CAD build for the part. Positions are in the model's coordinates, mm. A direction names the side the tool comes from. Coordinates: 2 decimals unless noted, no trailing zeros. Write each loop counter-clockwise with the first axis right and the second up, starting at its lowest first coordinate (ties: lowest second). Pieces come first, ordered by that corner, then holes. Notation, with made-up numbers: M 60,48 L 67,48 A16 ccw 67,78 Z; hole C -31.75,67 d2. An arc over 180 degrees is marked long. Put each result on its own line as item: value. Start each with the question number.
```python
from build123d import *

# Parameters (mm, degrees)
F0_R          = 13
F1_DEPTH      = 6
F2_R          = 10.5
F3_DEPTH      = 19
F3_DEPTH_BACK = 110
F6_START      = -19
F5_R          = 11.5
F5_R_2        = 10.5
F6_DEPTH      = 3
F8_START      = -15
F7_R          = 12.5
F7_R_2        = 10.5
F8_DEPTH      = 4
F10_DEPTH     = 5
F11_R         = 4.5
F12_DEPTH     = 153


with BuildPart() as f1:
    # F0 (on Front) → F1 (new body)
    with BuildSketch(Plane.XZ):
        Circle(F0_R)
    extrude(amount=F1_DEPTH)

    # F2 (on face) → F3 (join, two sides)
    with BuildSketch(Plane.XZ.offset(6)) as f3_sk:
        Circle(F2_R)
    extrude(amount=F3_DEPTH)
    extrude(f3_sk.sketch, amount=-F3_DEPTH_BACK)

    # F5 (on face) → F6 (join)
    with BuildSketch(Plane(origin=(0, 104, 0), x_dir=(-1, 0, 0), z_dir=(0, 1, 0)).offset(F6_START)):
        Circle(F5_R)
        Circle(F5_R_2, mode=Mode.SUBTRACT)
    extrude(amount=-F6_DEPTH)

    # F7 (on face) → F8 (join)
    with BuildSketch(Plane(origin=(0, 104, 0), x_dir=(-1, 0, 0), z_dir=(0, 1, 0)).offset(F8_START)):
        Circle(F7_R)
        Circle(F7_R_2, mode=Mode.SUBTRACT)
    extrude(amount=-F8_DEPTH)

    # F9 (on face) → F10 (join)
    with BuildSketch(Plane.XZ.offset(25)):
        Polygon((9.3875564858, -3.3022610956), (7.5536202416, 6.4787318484), (-1.8339362442, 9.780992944), (-9.3875564858, 3.3022610956), (-7.5536202416, -6.4787318484), (1.8339362442, -9.780992944), align=None)
    extrude(amount=F10_DEPTH)

    # F11 (on face) → F12 (cut)
    with BuildSketch(Plane.XZ.offset(30)):
        Circle(F11_R)
    extrude(amount=-F12_DEPTH, mode=Mode.SUBTRACT)


solid = f1.part
```
(1) Slice it at B-B, the plane y = 66.5. Write the cut outline in (x, z).
(2) Two-plate mould, pull along Y, no slides. Class faces 5 (the face through (4.04, -30, 2.31)), 6 (the face through (-3.4, 82, -10.2)), 7 (the face through (-10.316, -2.958, -7.91)): +Y half, -Y half, draft (parallel to the pull), parting line (faces both ways), or undercut.
(3) Which spindle directions (+Z, -Z, +X, -X, +Y, -Y) get a long thin tool onto all of the face, cutting with end or side? Do faces 1 (the face through (10, 40.4, 3.2)), 2 (the face through (5.558, -27.465, -6.587)), 3 (the face through (-5.558, -27.465, 6.587)), 4 (the face through (4, -25, 8)). Say none if no direction does.
(4) Drop flat-ended pins along their axis: pin 1 (5.5 mm diameter, centred on x = 0, z = 0, fed in from -Y); pin 2 (4 mm diameter, centred on x = 9, y = 49.5, fed in from -Z); pin 3 (4 mm diameter, centred on x = -4.5, y = 29.5, fed in from +Z); pin 4 (4 mm diameter, centred on y = 48.5, z = -8.5, fed in from +X). Give the stop position or say it passes through.
(5) Slice it at D-D, the plane y = 87.5. Write the cut outline in (x, z), then the cut area to 3 significant figures.
(6) Drill centre lines: line 1 (Z direction, x = 0, y = 41.5); line 2 (Y direction, x = -11.25, z = 3.25); line 3 (X direction, y = 59, z = 2.25). Where is each one in solid material? Low to high. Write a range as [from, to].
Result set:
1. outline: C 0,0 d21; hole C 0,0 d9
2. face 5: -Y half
2. face 6: undercut
2. face 7: draft
3. face 1: none
3. face 2: -Z, +X, -Y
3. face 3: +Z, -X, -Y
3. face 4: -Y
4. pin 1: passes through
4. pin 2: stops at z = -7.83
4. pin 3: stops at z = 10.2
4. pin 4: stops at x = 8.25
5. outline: C 0,0 d25; hole C 0,0 d9
5. area: 427 mm^2
6. line 1: z = [-10.5, -4.5], [4.5, 10.5]
6. line 2: y = [-6, 0], [85, 89]
6. line 3: x = [-10.26, -3.9], [3.9, 10.26]
